Work out the finished part from the listing and answer in its coordinate system (mm). Face numbers are marked on the shaded views. Coordinates: 2 decimals unless noted, no trailing zeros. Write each loop counter-clockwise with the first axis right and the second up, starting at its lowest first coordinate (ties: lowest second). Pieces come first, ordered by that corner, then holes. Notation, with made-up numbers: (2.5, 79.5) - (21.5, 79.5) arc R30 ccw to (21.5, 114.5) - close; hole circle Ø7 at (47.5, 21.25). An arc over 180 degrees is marked (long way). One line per item, written item: value.
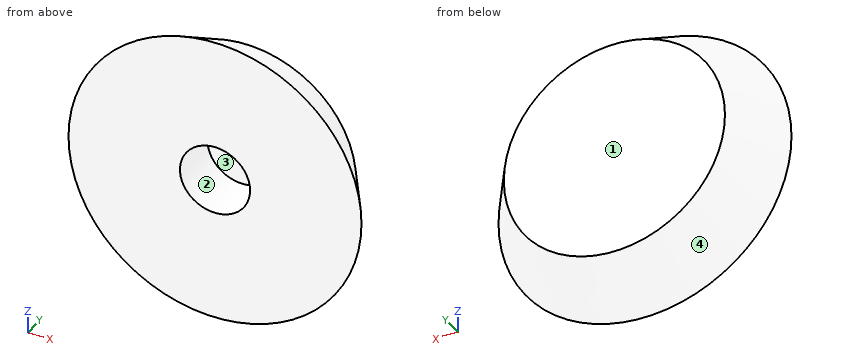
```python
from build123d import *

# Parameters (mm, degrees)
IZIM2_R                     = 5.095961834
IZIM2_R_2                   = 2.44
Y_KSEKLIK_EKSTR_ZYON1_DEPTH = 2
Y_KSEKLIK_EKSTR_ZYON1_TAPER = 32
IZIM3_R                     = 3.44
IZIM3_R_2                   = 2.44
EKSTR_ZYON_NCE1_DEPTH       = 2
IZIM4_R                     = 3.84622313
Y_KSEKLIK_EKSTR_ZYON2_DEPTH = 0.2
IZIM5_R                     = 2.44
IZIM5_R_2                   = 1.22
EKSTR_ZYON_NCE2_DEPTH       = 1.8


with BuildPart() as part:
    # Çizim2 → Yükseklik-Ekstrüzyon1 (new body)
    with BuildSketch(Plane(origin=(0, 0, 0), x_dir=(1, 0, 0), z_dir=(0, 1, 0))):
        Circle(IZIM2_R)
        Circle(IZIM2_R_2, mode=Mode.SUBTRACT)
    extrude(amount=Y_KSEKLIK_EKSTR_ZYON1_DEPTH, taper=Y_KSEKLIK_EKSTR_ZYON1_TAPER)

    # Çizim3 → Ekstrüzyon-İnce1 (add)
    with BuildSketch(Plane(origin=(0, 0, 0), x_dir=(1, 0, 0), z_dir=(0, 1, 0))):
        Circle(IZIM3_R)
        Circle(IZIM3_R_2, mode=Mode.SUBTRACT)
    extrude(amount=EKSTR_ZYON_NCE1_DEPTH)

    # Çizim4 → Yükseklik-Ekstrüzyon2 (add)
    with BuildSketch(Plane(origin=(0, 2, 0), x_dir=(1, 0, 0), z_dir=(0, 1, 0))):
        Circle(IZIM4_R)
    extrude(amount=-Y_KSEKLIK_EKSTR_ZYON2_DEPTH)

    # Çizim5 → Ekstrüzyon-İnce2 (add)
    with BuildSketch(Plane(origin=(0, 0, 0), x_dir=(1, 0, 0), z_dir=(0, 1, 0))):
        Circle(IZIM5_R)
        Circle(IZIM5_R_2, mode=Mode.SUBTRACT)
    extrude(amount=EKSTR_ZYON_NCE2_DEPTH)


solid = part.part
```
Item 1: Section D-D, the plane y = 1.35 is taken. Determine the outline of the cut face in (x, z).
Evaluation:
outline: circle Ø8.5 at (0, 0); hole circle Ø2.44 at (0, 0)
Item 2: Section B-B, the plane y = 0.7 is taken. Determine the outline of the cut face in (x, z), then the cut area to 3 significant figures.
Evaluation:
outline: circle Ø9.32 at (0, 0); hole circle Ø2.44 at (0, 0)
area: 63.5 mm2
Item 3: Consider probe 1 along X at (y, z) = (0.1, 0.5); probe 2 along Y at (x, z) = (-1, -0.5); probe 3 along X at (y, z) = (0.95, 0.25). Determine where each line is inside the solid, lowest interval first.
Evaluation:
probe 1: x = -5.01 to -1.11, 1.11 to 5.01
probe 2: y = 1.8 to 2
probe 3: x = -4.5 to -1.19, 1.19 to 4.5
Item 4: Section C-C, the plane z = 0 is taken. Give the number of separate pieces and of enclosed holes in the cut face, then the cut area to 3 significant figures.
Evaluation:
separate pieces: 1
enclosed holes: 2
area: 13.5 mm2
Item 5: Section A-A, the plane x = 0 is taken. Determine the outline of the cut face in (y, z).
Evaluation:
outline: (0, -5.1) - (2, -3.85) - (2, 3.85) - (0, 5.1) - (0, 1.22) - (1.8, 1.22) - (1.8, -1.22) - (0, -1.22) - close; hole (1.6, -3.44) - (1.8, -3.56) - (1.8, -3.44) - close; hole (1.6, 3.44) - (1.8, 3.44) - (1.8, 3.56) - close
Item 6: Given pin 1 (2 mm diameter, centred on x = 0, z = 0, fed in from -Y), flat-ended and moving along its own axis, determine where the tip first touches the part or whether it passes through.
Evaluation:
pin 1: stops at y = 1.8
Item 7: Determine the mould class of the marked faces 1, 2, 3 and 4 for opening direction X: +X half, -X half, draft (parallel to the pull), parting line (faces both ways), or undercut.
Evaluation:
face 1: draft
face 2: undercut
face 3: undercut
face 4: parting line
